from build123d import *

# Parameters (mm, degrees)
BOSS_EXTRUDE1_DEPTH      = 35.687
BOSS_EXTRUDE1_DEPTH_BACK = 35.687
SKETCH3_R                = 4.1656
CUT_EXTRUDE1_DEPTH       = 39.1
SKETCH5_R                = 4.1656
CUT_EXTRUDE2_DEPTH       = 39.1


with BuildPart() as part:
    # Sketch4 → Boss-Extrude1 (new body, two sides)
    with BuildSketch(Plane.XY) as boss_extrude1_sk:
        with BuildLine():
            Line((38.1, 0), (0, 0))
            Line((0, 0), (0, 38.1))
            ThreePointArc((0, 38.1), (4.490128061, 36.240128061), (6.35, 31.75))
            Line((6.35, 31.75), (6.35, 14.2748))
            ThreePointArc((6.35, 14.2748), (8.67112018, 8.67112018), (14.2748, 6.35))
            Line((14.2748, 6.35), (31.75, 6.35))
            ThreePointArc((31.75, 6.35), (36.240128061, 4.490128061), (38.1, 0))
        make_face()
    extrude(amount=BOSS_EXTRUDE1_DEPTH)
    extrude(boss_extrude1_sk.sketch, amount=-BOSS_EXTRUDE1_DEPTH_BACK)

    # Sketch3 → Cut-Extrude1 (cut, through all)
    with BuildSketch(Plane(origin=(0, 0, 0), x_dir=(1, 0, 0), z_dir=(0, 1, 0))):
        with Locations((19.05, -19.05)):
            Circle(SKETCH3_R)
        with Locations((19.05, 19.05)):
            Circle(SKETCH3_R)
    extrude(amount=CUT_EXTRUDE1_DEPTH, mode=Mode.SUBTRACT)

    # Sketch5 → Cut-Extrude2 (cut, through all)
    with BuildSketch(Plane(origin=(0, 0, 0), x_dir=(0, 0, -1), z_dir=(1, 0, 0))):
        with Locations((-19.05, 19.05)):
            Circle(SKETCH5_R)
        with Locations((19.05, 19.05)):
            Circle(SKETCH5_R)
    extrude(amount=CUT_EXTRUDE2_DEPTH, mode=Mode.SUBTRACT)


solid = part.part
Read the model definition and answer for the solid it produces. Units are mm, in the model's axes. A direction names the side the tool comes from. Give positions to 0.01 mm unless a question says otherwise; leave off trailing zeros. Write each loop counter-clockwise with the first axis right and the second up, starting at its lowest first coordinate (ties: lowest second). Pieces come first, ordered by that corner, then holes. Notation, with made-up numbers: (85.25, -7) - (91.25, -7) arc R28 cw to (91.25, 11) - close; hole circle Ø3 at (-14, -3.5). An arc over 180 degrees is marked (long way). Use CSV: the item, a comma, the result in double quotes. Start each with the question number.
Item 1: The part is cut by section D-D, the plane z = -30. Give the vertices of the cut face in (x, y), and give its area (3 significant figures).
Item 2: The mould has two halves that part along Z. Classify faces 1 (the flat face through (19, 0, 0)), 2 (the cylindrical face through (18.51, 3.13, 14.92)), 3 (the flat face through (11, 6, 35.687)): pulls with the +Z half, pulls with the -Z half, needs draft (parallel to the pull), parting line crosses it, or undercut.
Item 3: Flat-ended cylindrical pins translate along their axes: P1, Ø5, axis at y = 19.05, z = 19.05, coming from the +X side; P2, Ø8.5, axis at y = 19, z = 2, coming from the +X side; P3, Ø8, axis at y = 17, z = -17.5, coming from the +X side; P4, Ø5, axis at x = 26.5, z = -10.5, coming from the +Y side. Find the tip coordinate at first contact, or state that the pin passes through.
Item 4: For faces 4 (the flat face through (6.35, 23, 0)), 5 (the flat face through (11, 6, -35.687)), determine the directions among +Z, -Z, +X, -X, +Y, -Y from which every point of the face is accessible in a straight line to the end or side of a thin tool.
Item 5: The part is cut by section B-B, the plane z = 19.05. Give the vertices of the cut face in (x, y).
Item 6: Consider line 1 (Z direction, x = 1.5, y = 19.05); line 2 (Y direction, x = 32, z = -4); line 3 (X direction, y = 3.5, z = -19.05). Determine where each line is inside the solid, lowest interval first.
Item 7: The part is cut by section A-A, the plane x = 19.05. Give the vertices of the cut face in (y, z), and give its area (3 significant figures).
Taken from the geometry:
1,outline,"(0, 0) - (38.1, 0) arc R6.35 ccw to (31.75, 6.35) - (14.27, 6.35) arc R7.92 cw to (6.35, 14.27) - (6.35, 31.75) arc R6.35 ccw to (0, 38.1) - close"
1,area,"440 mm2"
2,face 1,"needs draft"
2,face 2,"undercut"
2,face 3,"pulls with the +Z half"
3,P1,"through"
3,P2,"x = 6.35"
3,P3,"x = 6.45"
3,P4,"y = 6.35"
4,face 4,"+Z, -Z, +X, +Y"
4,face 5,"-Z, +X, -X, +Y, -Y"
5,outline,"(0, 0) - (14.88, 0) - (14.88, 6.35) - (14.27, 6.35) arc R7.92 cw to (6.35, 14.27) - (6.35, 14.88) - (0, 14.88) - close; (0, 23.22) - (6.35, 23.22) - (6.35, 31.75) arc R6.35 ccw to (0, 38.1) - close; (23.22, 0) - (38.1, 0) arc R6.35 ccw to (31.75, 6.35) - (23.22, 6.35) - close"
6,line 1,"-35.69 to -23.22, -14.88 to 14.88, 23.22 to 35.69"
6,line 2,"0 to 6.35"
6,line 3,"0 to 14.88, 23.22 to 37.05"
7,outline,"(0, -35.69) - (6.35, -35.69) - (6.35, -23.22) - (0, -23.22) - close; (0, -14.88) - (6.35, -14.88) - (6.35, 14.88) - (0, 14.88) - close; (0, 23.22) - (6.35, 23.22) - (6.35, 35.69) - (0, 35.69) - close"
7,area,"347 mm2"
